The listing builds one solid part. Answer for the finished solid, in the listing's coordinates (mm). Face numbers are marked on the shaded views. A direction names the side the tool comes from. Give positions to 0.01 mm unless a question says otherwise; leave off trailing zeros. Write each loop counter-clockwise with the first axis right and the second up, starting at its lowest first coordinate (ties: lowest second). Pieces come first, ordered by that corner, then holes.
```python
from build123d import *

# Parameters (mm, degrees)
SKETCH1_W           = 11
SKETCH1_H           = 11
BOSS_EXTRUDE1_DEPTH = 9
SKETCH2_W           = 16
SKETCH2_H           = 13
BOSS_EXTRUDE2_DEPTH = 0.5
SKETCH3_R           = 2.446587027
BOSS_EXTRUDE3_DEPTH = 0.5


with BuildPart() as part:
    # Sketch1 → Boss-Extrude1 (new body)
    with BuildSketch(Plane(origin=(0, 0, 0), x_dir=(1, 0, 0), z_dir=(0, 1, 0))):
        with Locations((138.476530612, -102.126020408)):
            Rectangle(SKETCH1_W, SKETCH1_H)
    extrude(amount=BOSS_EXTRUDE1_DEPTH)

    # Sketch2 → Boss-Extrude2 (add)
    with BuildSketch(Plane.XZ):
        with Locations((138.476530612, 102.126020408)):
            Rectangle(SKETCH2_W, SKETCH2_H)
    extrude(amount=BOSS_EXTRUDE2_DEPTH)

    # Sketch3 → Boss-Extrude3 (add)
    with BuildSketch(Plane(origin=(0, 9, 0), x_dir=(1, 0, 0), z_dir=(0, 1, 0))):
        with Locations((138.476530612, -102.126020408)):
            Circle(SKETCH3_R)
    extrude(amount=BOSS_EXTRUDE3_DEPTH)


solid = part.part
```
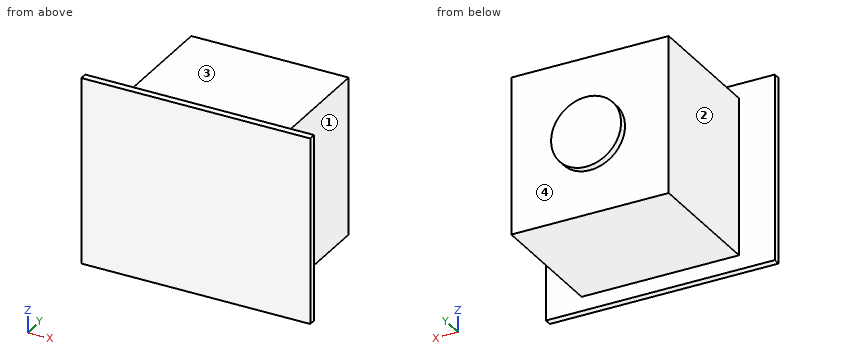
Item 1: A cutting plane is placed at D-D, the plane x = 134. Give the vertices of the cut face in (y, z), plus the area to 4 significant figures.
Conclusion:
outline: (-0.5, 95.63) - (0, 95.63) - (0, 96.63) - (9, 96.63) - (9, 107.63) - (0, 107.63) - (0, 108.63) - (-0.5, 108.63) - close
area: 105.5 mm2
Item 2: Each of these flat-tipped pins is pushed along its axis until it touches: P1, Ø5, axis at x = 135.5, y = 5.5, coming from the +Z side; P2, Ø2.5, axis at x = 139.5, y = 5, coming from the -Z side; P3, Ø2.5, axis at y = 3.5, z = 104.5, coming from the -X side. Where does it stop, or does it pass through?
Conclusion:
P1: stops at z = 107.63
P2: stops at z = 96.63
P3: stops at x = 132.98
Item 3: A cutting plane is placed at A-A, the plane x = 137.25. Give the vertices of the cut face in (y, z).
Conclusion:
outline: (-0.5, 95.63) - (0, 95.63) - (0, 96.63) - (9, 96.63) - (9, 100.01) - (9.5, 100.01) - (9.5, 104.24) - (9, 104.24) - (9, 107.63) - (0, 107.63) - (0, 108.63) - (-0.5, 108.63) - close
Item 4: Which of the six approach directions +Z, -Z, +X, -X, +Y, -Y give full straight-line access (tool end or side, diameter ignored) to the marked faces 1, 2, 3 and 4?
Conclusion:
face 1: +Z, -Z, +X, +Y
face 2: +Z, -Z, -X, +Y
face 3: +Z, +X, -X, +Y
face 4: +Y
Item 5: Consider probe 1 along Y at (x, z) = (133.5, 98.75); probe 2 along Y at (x, z) = (146, 101.25); probe 3 along Z at (x, y) = (135.25, 8.5). Determine where each line is inside the solid, lowest interval first.
Conclusion:
probe 1: y = -0.5 to 9
probe 2: y = -0.5 to 0
probe 3: z = 96.63 to 107.63
Item 6: A cutting plane is placed at C-C, the plane y = 7.75. Give the vertices of the cut face in (x, z).
Conclusion:
outline: (132.98, 96.63) - (143.98, 96.63) - (143.98, 107.63) - (132.98, 107.63) - close
Item 7: A cutting plane is placed at B-B, the plane z = 107. Give the vertices of the cut face in (x, y), plus the area to 3 significant figures.
Conclusion:
outline: (130.48, -0.5) - (146.48, -0.5) - (146.48, 0) - (143.98, 0) - (143.98, 9) - (132.98, 9) - (132.98, 0) - (130.48, 0) - close
area: 107 mm2
